Source: three-view drawing plus pictorial views. Frame: mm from the lowest corner of the part. A direction names the side the tool comes from. Round coordinates to 2 decimals unless told otherwise and drop trailing zeros. Loops run counter-clockwise (first coordinate to the right, second up) from the corner with the lowest first, then second, coordinate; pieces in that order, holes last. Notation, with made-up numbers: M 3,-17.5 L 50,-17.5 A25 cw 50,7.5 Z; hole C 83,78 d1. An arc over 180 degrees is marked long. Return JSON: item names as keys, results as strings. Group by question number.
1) Section C-C (y = 25.5). Output: boundary loops of the cut face in (x, z).
2) Access query for the marked faces 1, 2, 3, 4 and 5. Directions: +Z, -Z, +X, -X, +Y, -Y. A direction counts if a zero-diameter tool reaches every point of the face in a straight line with its end or side. Return the directions, or none.
3) Contact query for flat-ended pins moving along their axis: P1, Ø10, axis at x = 34, z = 15, coming from the +Y side; P2, Ø1.5, axis at x = 22.5, z = 15.5, coming from the +Y side; P3, Ø3.5, axis at x = 52, z = 14.5, coming from the -Y side; P4, Ø1.5, axis at y = 32, z = 8.5, coming from the -X side. Output: stop coordinate, or through.
4) Section B-B (x = 27). Output: boundary loops of the cut face in (y, z), plus the area to 3 significant figures.
5) Section A-A (x = 3). Output: boundary loops of the cut face in (y, z), plus the area to 3 significant figures.
6) Material intervals for line 1 (Z direction, x = 3, y = 28.75); line 2 (Y direction, x = 7.5, z = 4.5); line 3 (X direction, y = 5, z = 2.5), sorted ascending. Write a range as from..to.
7) Section D-D (x = 20). Output: boundary loops of the cut face in (y, z).
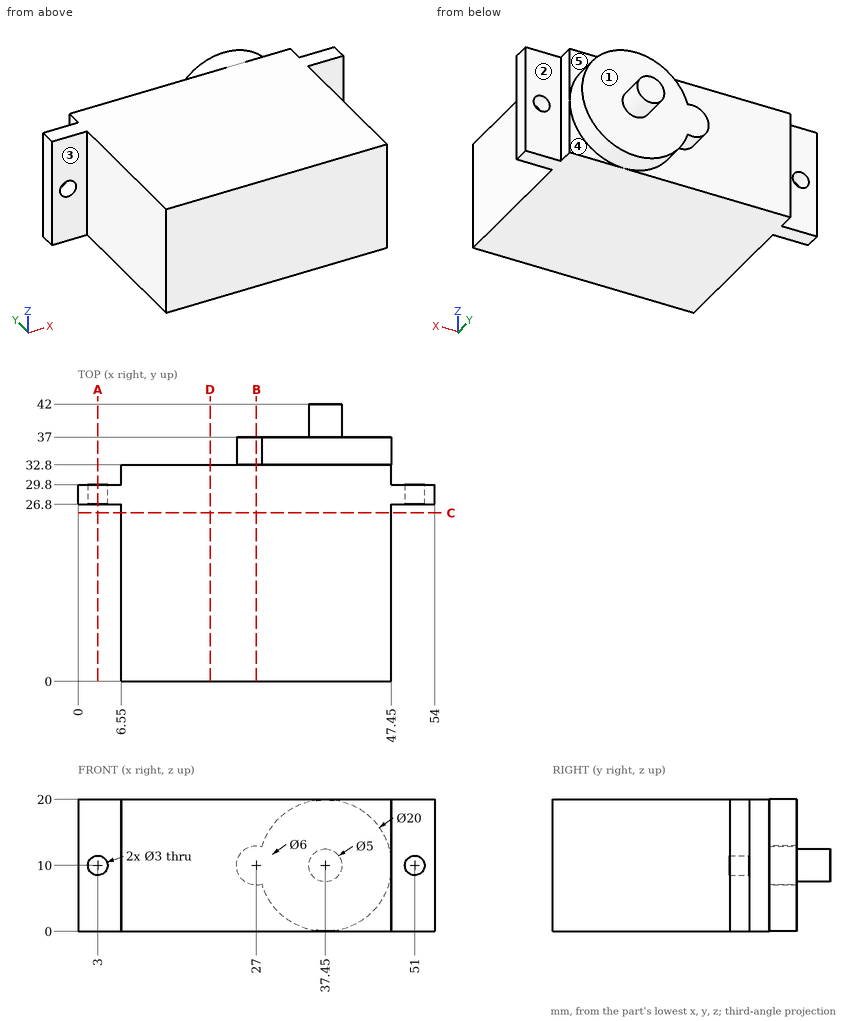
Returned:
{
 "1": {"outline": "M 6.55,0 L 47.45,0 L 47.45,20 L 6.55,20 Z"},
 "2": {"face 1": "+Y", "face 2": "+Z, -Z, +X, +Y", "face 3": "+Z, -Z, -X, -Y", "face 4": "-Z, +X, +Y", "face 5": "+Z, +X, +Y"},
 "3": {"P1": "stops at y = 42", "P2": "stops at y = 32.8", "P3": "stops at y = 26.8", "P4": "stops at x = 6.55"},
 "4": {"outline": "M 0,0 L 32.8,0 L 32.8,7 L 37,7 L 37,13 L 32.8,13 L 32.8,20 L 0,20 Z", "area": "681 mm^2"},
 "5": {"outline": "M 26.8,0 L 29.8,0 L 29.8,8.5 L 26.8,8.5 Z; M 26.8,11.5 L 29.8,11.5 L 29.8,20 L 26.8,20 Z", "area": "51.0 mm^2"},
 "6": {"line 1": "z = 0..8.5, 11.5..20", "line 2": "y = 0..32.8", "line 3": "x = 6.55..47.45"},
 "7": {"outline": "M 0,0 L 32.8,0 L 32.8,20 L 0,20 Z"}
}
